from build123d import *

# Parameters (mm, degrees)
BOSS_EXTRUDE1_DEPTH = 17.5
CHAMFER1_SIZE       = 5


with BuildPart() as part:
    # Sketch1 → Boss-Extrude1 (new, symmetric)
    with BuildSketch(Plane.XY):
        with BuildLine():
            Line((-100, 0), (-80, 0))
            ThreePointArc((-80, 0), (-76.464466094, 1.464466094), (-75, 5))
            Line((-75, 5), (-75, 30))
            ThreePointArc((-75, 30), (-72.071067812, 37.071067812), (-65, 40))
            Line((-65, 40), (65, 40))
            ThreePointArc((65, 40), (72.071067812, 37.071067812), (75, 30))
            Line((75, 30), (75, 5))
            ThreePointArc((75, 5), (76.464466094, 1.464466094), (80, 0))
            Line((80, 0), (100, 0))
            Line((100, 0), (100, -4))
            Line((100, -4), (76, -4))
            ThreePointArc((76, -4), (72.464466094, -2.535533906), (71, 1))
            Line((71, 1), (71, 30))
            ThreePointArc((71, 30), (69.242640687, 34.242640687), (65, 36))
            Line((65, 36), (-65, 36))
            ThreePointArc((-65, 36), (-69.242640687, 34.242640687), (-71, 30))
            Line((-71, 30), (-71, 1))
            ThreePointArc((-71, 1), (-72.464466094, -2.535533906), (-76, -4))
            Line((-76, -4), (-100, -4))
            Line((-100, -4), (-100, 0))
        make_face()
    extrude(amount=BOSS_EXTRUDE1_DEPTH, both=True)

    # Chamfer1
    # the kernel refuses this chamfer: 5 mm, written as the material it takes off along each edge
    with BuildSketch(Plane(origin=(-100, 0, 30.35841494), x_dir=(0.9996219169112968, 0.027495876610586334, 0), z_dir=(0, 0, -1)), Plane(origin=(100, 0, 30.35841494), x_dir=(0.0274958766105877, -0.9996219169112968, 0), z_dir=(0, 0, -1))) as chamfer1_piece_1:
        Polygon((CHAMFER1_SIZE * 0.999621916911, CHAMFER1_SIZE * 0.0274958766106), (-CHAMFER1_SIZE * 0.0274958766106, CHAMFER1_SIZE * 0.999621916911), (0, 0), align=None)
    extrude(amount=60.71682988, mode=Mode.SUBTRACT)


solid = part.part
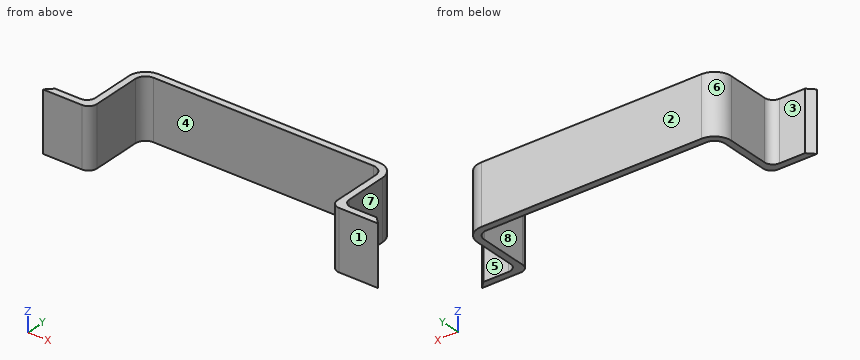
Input: part model. Units: mm. Frame: model coordinates. Face numbers are marked on the shaded views. A direction names the side the tool comes from. Give positions to 0.01 mm unless a question says otherwise; leave off trailing zeros. Order: outer loops, then holes, each group sorted by start corner. A loop starts at its lowest first (then second) coordinate and runs counter-clockwise, first axis right, second up. Notation, with made-up numbers: M 6.5,88 L 55.5,88 A13 cw 55.5,111 Z; hole C -4.5,23.5 d9. An arc over 180 degrees is marked long. Answer as a JSON object with one key per item and string values.
1. Cut plane D-D, the plane x = -32. Output: boundary loops of the cut face in (y, z).
Result sheet:
{"outline": "M 36,-17.5 L 40,-17.5 L 40,17.5 L 36,17.5 Z"}
2. Cut plane A-A, the plane y = 22. Output: boundary loops of the cut face in (x, z).
Result sheet:
{"outline": "M -75,-17.5 L -71,-17.5 L -71,17.5 L -75,17.5 Z; M 71,-17.5 L 75,-17.5 L 75,17.5 L 71,17.5 Z"}
3. Pull-direction query (X, two-part tool) for the marked faces 6, 7 and 8; classes: +X half, -X half, draft (parallel to the pull), parting line (faces both ways), or undercut.
Result sheet:
{"face 6": "-X half", "face 7": "+X half", "face 8": "undercut"}
4. Cut plane B-B, the plane z = -13. Output: boundary loops of the cut face in (x, y), and give its area (3 significant figures).
Result sheet:
{"outline": "M -99,-4 L -76,-4 A5 ccw -71,1 L -71,30 A6 cw -65,36 L 65,36 A6 cw 71,30 L 71,1 A5 ccw 76,-4 L 99,-4 L 95,0 L 80,0 A5 cw 75,5 L 75,30 A10 ccw 65,40 L -65,40 A10 ccw -75,30 L -75,5 A5 cw -80,0 L -95,0 Z", "area": "1,070 mm²"}
5. Reachability of the marked faces 1, 2, 3, 4 and 5 from +Z, -Z, +X, -X, +Y, -Y: full face, straight path, thin tool, end or side. Return the list, or none.
Result sheet:
{"face 1": "+Z, -Z, +X, -X, -Y", "face 2": "+Z, -Z, +X, -X, +Y", "face 3": "+Z, -Z, -X, +Y", "face 4": "+Z, -Z, -Y", "face 5": "+Z, -Z, +X, +Y"}
6. Cut plane C-C, the plane y = 34. Output: boundary loops of the cut face in (x, z).
Result sheet:
{"outline": "M -74.17,-17.5 L -69.47,-17.5 L -69.47,17.5 L -74.17,17.5 Z; M 69.47,-17.5 L 74.17,-17.5 L 74.17,17.5 L 69.47,17.5 Z"}
7. First-contact query: P1, Ø14.5, axis at y = 19, z = -4.5, coming from the +X side; P2, Ø12, axis at x = 36.5, y = 34, coming from the +Z side; P3, Ø16.5, axis at x = -85.5, z = -7.5, coming from the +Y side; P4, Ø16.5, axis at x = 85, z = 2, coming from the +Y side. Flat tips, straight axial feed; report the tip coordinate or a pass-through.
Result sheet:
{"P1": "x = 75", "P2": "z = 17.5", "P3": "y = 0.82", "P4": "y = 1.2"}
8. Ray query, line 1 (X direction, y = 21, z = 0.5); line 2 (Y direction, x = -32, z = 13); line 3 (X direction, y = 31, z = -1). Return the intervals inside material, ascending. Write a range as [from, to].
Result sheet:
{"line 1": "[-75, -71], [71, 75]", "line 2": "[36, 40]", "line 3": "[-74.95, -70.92], [70.92, 74.95]"}
